The listing builds one solid part. Answer for the finished solid, in the listing's coordinates (mm). A direction names the side the tool comes from. Round coordinates to 2 decimals unless told otherwise and drop trailing zeros. Write each loop counter-clockwise with the first axis right and the second up, starting at its lowest first coordinate (ties: lowest second). Pieces come first, ordered by that corner, then holes. Notation, with made-up numbers: (49.5, 55) - (103.5, 55) arc R14 ccw to (103.5, 81) - close; hole circle Ø5 at (-6, 27). An arc over 180 degrees is marked (long way). Return JSON: item names as keys, results as strings. Group by question number.
(1) Determine the mould class of faces 1 (the cylindrical face through (16.29, 5.9, 21.19)), 2 (the cylindrical face through (34.166, 6.345, 3.318)), 3 (the flat face through (-45, -9.752, 13)) for opening direction X: +X half, -X half, draft (parallel to the pull), parting line (faces both ways), or undercut.
(2) Find the intervals of material crossed by line 1 along Z through (x, y) = (-22, 0); line 2 along Y through (x, z) = (11.5, 7); line 3 along Z through (x, y) = (-102, -3), in increasing order. Write a range as [from, to].
(3) Which of the six approach directions +Z, -Z, +X, -X, +Y, -Y give full straight-line access (tool end or side, diameter ignored) to faces 4 (the flat face through (22, 6, 19.05)), 5 (the flat face through (32, 6, 19.05)), 6 (the cylindrical face through (-42.768, 19.825, 2.291))?
(4) Section C-C, the plane z = 2.75 is taken. Write down the section's boundary in (x, y), then the cut area to 3 significant figures.
(5) Section B-B, the plane x = -35 is taken. Write down the section's boundary in (y, z), then the cut area to 3 significant figures.
(6) Each of these flat-tipped pins is pushed along its axis until it touches: pin 1 (6 mm diameter, centred on x = -107, y = 13.5, fed in from +Z); pin 2 (1 mm diameter, centred on x = 10.5, y = 3, fed in from +Z); pin 3 (6.5 mm diameter, centred on x = -2, y = 7.5, fed in from +Z); pin 4 (6.5 mm diameter, centred on x = -36, y = -1.5, fed in from +Z). Where does it stop, or does it pass through?
```python
from build123d import *

# Parameters (mm, degrees)
F0_W          = 158.75
F0_H          = 31.75
F1_DEPTH      = 19.05
F3_R          = 7.62
F2_R          = 1.905
F4_DEPTH      = 21.9981725439
F4_DEPTH_BACK = 9.7518274561


with BuildPart() as f1:
    # F0 (on Top) → F1 (new body)
    with BuildSketch(Plane.XY):
        with Locations((-43.8790681958, 6.1231725439)):
            Rectangle(F0_W, F0_H)
    extrude(amount=F1_DEPTH)

    # F3
    f3_edges = [f1.edges().sort_by_distance(p)[0] for p in [
        (-43.879068, 21.998173, 0),
        (-123.254068, 6.123173, 0),
        (-43.879068, -9.751827, 0),
        (35.495932, 6.123173, 0),
    ]]
    fillet(f3_edges, radius=F3_R)

    # F2 (on Front) → F4 (join, two sides)
    with BuildSketch(Plane.XZ) as f4_sk:
        with Locations((-105.110168457, 19.2852988839)):
            Circle(F2_R)
        with Locations((-92.5481468439, 19.2852988839)):
            Circle(F2_R)
        with Locations((-78.6401927471, 19.2852988839)):
            Circle(F2_R)
        with Locations((-66.7505128102, 19.2852988839)):
            Circle(F2_R)
        with Locations((-54.8614611642, 19.2852988839)):
            Circle(F2_R)
        with Locations((-43.4210499542, 19.2852988839)):
            Circle(F2_R)
        with Locations((-31.7563166635, 19.2852988839)):
            Circle(F2_R)
        with Locations((-18.9705938101, 19.2852988839)):
            Circle(F2_R)
        with Locations((-6.8572163582, 19.2852988839)):
            Circle(F2_R)
        with Locations((-118.1202022152, 19.2852988839)):
            Circle(F2_R)
        with Locations((5.2561564371, 19.2852988839)):
            Circle(F2_R)
        with Locations((16.2479281425, 19.2852988839)):
            Circle(F2_R)
        with Locations((27.4640191346, 19.2852988839)):
            Circle(F2_R)
    extrude(amount=-F4_DEPTH)
    extrude(f4_sk.sketch, amount=F4_DEPTH_BACK)


solid = f1.part
```
Working result:
{
 "1": {"face 1": "undercut", "face 2": "+X half", "face 3": "draft"},
 "2": {"line 1": "z = [0, 19.05]", "line 2": "y = [-9.73, 21.97]", "line 3": "z = [0.05, 19.05]"},
 "3": {"face 4": "+Z, +Y, -Y", "face 5": "+Z, +X, +Y, -Y", "face 6": "-Z, +X, -X, +Y"},
 "4": {"outline": "(-121.49, -7.99) - (33.74, -7.99) - (33.74, 20.24) - (-121.49, 20.24) - close", "area": "4,380 mm^2"},
 "5": {"outline": "(-9.75, 7.62) arc R7.62 ccw to (-2.13, 0) - (14.38, 0) arc R7.62 ccw to (22, 7.62) - (22, 19.05) - (-9.75, 19.05) - close", "area": "580 mm^2"},
 "6": {"pin 1": "stops at z = 21.19", "pin 2": "stops at z = 19.05", "pin 3": "stops at z = 20.31", "pin 4": "stops at z = 20.91"}
}
